Geometry: final body of the model. Coordinates: model frame, mm. Give positions to 0.01 mm unless a question says otherwise; leave off trailing zeros. Loops run counter-clockwise (first coordinate to the right, second up) from the corner with the lowest first, then second, coordinate; pieces in that order, holes last.
from build123d import *

# Parameters (mm, degrees)
SKETCH23_R          = 70.65
SKETCH23_R_2        = 14
BOSS_EXTRUDE3_DEPTH = 10
LO_BAT_HOP_SO_REACH = 12
SKETCH24_R          = 4
SKETCH24_R_2        = 6.25


with BuildPart() as part:
    # Sketch23 → Boss-Extrude3 (new body)
    with BuildSketch(Plane(origin=(0, 0, 0), x_dir=(1, 0, 0), z_dir=(0, 1, 0))):
        Polygon((106, -490.925019631), (106, 0), (79.205080757, 100), (-79.205080757, 100), (-106, 0), (-106, -490.925019631), (-20, -601), (20, -601), align=None)
        Circle(SKETCH23_R, mode=Mode.SUBTRACT)
        with Locations((0, -330)):
            Circle(SKETCH23_R_2, mode=Mode.SUBTRACT)
    extrude(amount=BOSS_EXTRUDE3_DEPTH)

    # Sketch24 → lo bat hop so (cut, up to next)
    with BuildSketch(Plane(origin=(0, 10, 0), x_dir=(1, 0, 0), z_dir=(0, 1, 0)), mode=Mode.PRIVATE) as lo_bat_hop_so_sk1:
        with Locations((-83, -150)):
            Circle(SKETCH24_R)
    lo_bat_hop_so_tool1 = extrude(lo_bat_hop_so_sk1.sketch, amount=-LO_BAT_HOP_SO_REACH, mode=Mode.PRIVATE) & part.part
    add(lo_bat_hop_so_tool1.solids().sort_by_distance((-83, 10, 150))[0], mode=Mode.SUBTRACT)
    # Sketch24 → lo bat hop so (cut, up to next)
    with BuildSketch(Plane(origin=(0, 10, 0), x_dir=(1, 0, 0), z_dir=(0, 1, 0)), mode=Mode.PRIVATE) as lo_bat_hop_so_sk2:
        with Locations((-83, -388)):
            Circle(SKETCH24_R)
    lo_bat_hop_so_tool2 = extrude(lo_bat_hop_so_sk2.sketch, amount=-LO_BAT_HOP_SO_REACH, mode=Mode.PRIVATE) & part.part
    add(lo_bat_hop_so_tool2.solids().sort_by_distance((-83, 10, 388))[0], mode=Mode.SUBTRACT)
    # Sketch24 → lo bat hop so (cut, up to next)
    with BuildSketch(Plane(origin=(0, 10, 0), x_dir=(1, 0, 0), z_dir=(0, 1, 0)), mode=Mode.PRIVATE) as lo_bat_hop_so_sk3:
        with Locations((83, -388)):
            Circle(SKETCH24_R)
    lo_bat_hop_so_tool3 = extrude(lo_bat_hop_so_sk3.sketch, amount=-LO_BAT_HOP_SO_REACH, mode=Mode.PRIVATE) & part.part
    add(lo_bat_hop_so_tool3.solids().sort_by_distance((83, 10, 388))[0], mode=Mode.SUBTRACT)
    # Sketch24 → lo bat hop so (cut, up to next)
    with BuildSketch(Plane(origin=(0, 10, 0), x_dir=(1, 0, 0), z_dir=(0, 1, 0)), mode=Mode.PRIVATE) as lo_bat_hop_so_sk4:
        with Locations((83, -150)):
            Circle(SKETCH24_R)
    lo_bat_hop_so_tool4 = extrude(lo_bat_hop_so_sk4.sketch, amount=-LO_BAT_HOP_SO_REACH, mode=Mode.PRIVATE) & part.part
    add(lo_bat_hop_so_tool4.solids().sort_by_distance((83, 10, 150))[0], mode=Mode.SUBTRACT)
    # Sketch24 → lo bat hop so (cut, up to next)
    with BuildSketch(Plane(origin=(0, 10, 0), x_dir=(1, 0, 0), z_dir=(0, 1, 0)), mode=Mode.PRIVATE) as lo_bat_hop_so_sk5:
        with Locations((-83, -20)):
            Circle(SKETCH24_R)
    lo_bat_hop_so_tool5 = extrude(lo_bat_hop_so_sk5.sketch, amount=-LO_BAT_HOP_SO_REACH, mode=Mode.PRIVATE) & part.part
    add(lo_bat_hop_so_tool5.solids().sort_by_distance((-83, 10, 20))[0], mode=Mode.SUBTRACT)
    # Sketch24 → lo bat hop so (cut, up to next)
    with BuildSketch(Plane(origin=(0, 10, 0), x_dir=(1, 0, 0), z_dir=(0, 1, 0)), mode=Mode.PRIVATE) as lo_bat_hop_so_sk6:
        with Locations((83, -20)):
            Circle(SKETCH24_R)
    lo_bat_hop_so_tool6 = extrude(lo_bat_hop_so_sk6.sketch, amount=-LO_BAT_HOP_SO_REACH, mode=Mode.PRIVATE) & part.part
    add(lo_bat_hop_so_tool6.solids().sort_by_distance((83, 10, 20))[0], mode=Mode.SUBTRACT)
    # Sketch24 → lo bat hop so (cut, up to next)
    with BuildSketch(Plane(origin=(0, 10, 0), x_dir=(1, 0, 0), z_dir=(0, 1, 0)), mode=Mode.PRIVATE) as lo_bat_hop_so_sk7:
        with Locations((-70, -380)):
            Circle(SKETCH24_R_2)
    lo_bat_hop_so_tool7 = extrude(lo_bat_hop_so_sk7.sketch, amount=-LO_BAT_HOP_SO_REACH, mode=Mode.PRIVATE) & part.part
    add(lo_bat_hop_so_tool7.solids().sort_by_distance((-70, 10, 380))[0], mode=Mode.SUBTRACT)
    # Sketch24 → lo bat hop so (cut, up to next)
    with BuildSketch(Plane(origin=(0, 10, 0), x_dir=(1, 0, 0), z_dir=(0, 1, 0)), mode=Mode.PRIVATE) as lo_bat_hop_so_sk8:
        with Locations((-70, -300)):
            Circle(SKETCH24_R_2)
    lo_bat_hop_so_tool8 = extrude(lo_bat_hop_so_sk8.sketch, amount=-LO_BAT_HOP_SO_REACH, mode=Mode.PRIVATE) & part.part
    add(lo_bat_hop_so_tool8.solids().sort_by_distance((-70, 10, 300))[0], mode=Mode.SUBTRACT)
    # Sketch24 → lo bat hop so (cut, up to next)
    with BuildSketch(Plane(origin=(0, 10, 0), x_dir=(1, 0, 0), z_dir=(0, 1, 0)), mode=Mode.PRIVATE) as lo_bat_hop_so_sk9:
        with Locations((-70, -210)):
            Circle(SKETCH24_R_2)
    lo_bat_hop_so_tool9 = extrude(lo_bat_hop_so_sk9.sketch, amount=-LO_BAT_HOP_SO_REACH, mode=Mode.PRIVATE) & part.part
    add(lo_bat_hop_so_tool9.solids().sort_by_distance((-70, 10, 210))[0], mode=Mode.SUBTRACT)
    # Sketch24 → lo bat hop so (cut, up to next)
    with BuildSketch(Plane(origin=(0, 10, 0), x_dir=(1, 0, 0), z_dir=(0, 1, 0)), mode=Mode.PRIVATE) as lo_bat_hop_so_sk10:
        with Locations((-70, -150)):
            Circle(SKETCH24_R_2)
    lo_bat_hop_so_tool10 = extrude(lo_bat_hop_so_sk10.sketch, amount=-LO_BAT_HOP_SO_REACH, mode=Mode.PRIVATE) & part.part
    add(lo_bat_hop_so_tool10.solids().sort_by_distance((-70, 10, 150))[0], mode=Mode.SUBTRACT)
    # Sketch24 → lo bat hop so (cut, up to next)
    with BuildSketch(Plane(origin=(0, 10, 0), x_dir=(1, 0, 0), z_dir=(0, 1, 0)), mode=Mode.PRIVATE) as lo_bat_hop_so_sk11:
        with Locations((-70, -90)):
            Circle(SKETCH24_R_2)
    lo_bat_hop_so_tool11 = extrude(lo_bat_hop_so_sk11.sketch, amount=-LO_BAT_HOP_SO_REACH, mode=Mode.PRIVATE) & part.part
    add(lo_bat_hop_so_tool11.solids().sort_by_distance((-70, 10, 90))[0], mode=Mode.SUBTRACT)
    # Sketch24 → lo bat hop so (cut, up to next)
    with BuildSketch(Plane(origin=(0, 10, 0), x_dir=(1, 0, 0), z_dir=(0, 1, 0)), mode=Mode.PRIVATE) as lo_bat_hop_so_sk12:
        with Locations((70, -90)):
            Circle(SKETCH24_R_2)
    lo_bat_hop_so_tool12 = extrude(lo_bat_hop_so_sk12.sketch, amount=-LO_BAT_HOP_SO_REACH, mode=Mode.PRIVATE) & part.part
    add(lo_bat_hop_so_tool12.solids().sort_by_distance((70, 10, 90))[0], mode=Mode.SUBTRACT)
    # Sketch24 → lo bat hop so (cut, up to next)
    with BuildSketch(Plane(origin=(0, 10, 0), x_dir=(1, 0, 0), z_dir=(0, 1, 0)), mode=Mode.PRIVATE) as lo_bat_hop_so_sk13:
        with Locations((70, -150)):
            Circle(SKETCH24_R_2)
    lo_bat_hop_so_tool13 = extrude(lo_bat_hop_so_sk13.sketch, amount=-LO_BAT_HOP_SO_REACH, mode=Mode.PRIVATE) & part.part
    add(lo_bat_hop_so_tool13.solids().sort_by_distance((70, 10, 150))[0], mode=Mode.SUBTRACT)
    # Sketch24 → lo bat hop so (cut, up to next)
    with BuildSketch(Plane(origin=(0, 10, 0), x_dir=(1, 0, 0), z_dir=(0, 1, 0)), mode=Mode.PRIVATE) as lo_bat_hop_so_sk14:
        with Locations((70, -210)):
            Circle(SKETCH24_R_2)
    lo_bat_hop_so_tool14 = extrude(lo_bat_hop_so_sk14.sketch, amount=-LO_BAT_HOP_SO_REACH, mode=Mode.PRIVATE) & part.part
    add(lo_bat_hop_so_tool14.solids().sort_by_distance((70, 10, 210))[0], mode=Mode.SUBTRACT)
    # Sketch24 → lo bat hop so (cut, up to next)
    with BuildSketch(Plane(origin=(0, 10, 0), x_dir=(1, 0, 0), z_dir=(0, 1, 0)), mode=Mode.PRIVATE) as lo_bat_hop_so_sk15:
        with Locations((70, -300)):
            Circle(SKETCH24_R_2)
    lo_bat_hop_so_tool15 = extrude(lo_bat_hop_so_sk15.sketch, amount=-LO_BAT_HOP_SO_REACH, mode=Mode.PRIVATE) & part.part
    add(lo_bat_hop_so_tool15.solids().sort_by_distance((70, 10, 300))[0], mode=Mode.SUBTRACT)
    # Sketch24 → lo bat hop so (cut, up to next)
    with BuildSketch(Plane(origin=(0, 10, 0), x_dir=(1, 0, 0), z_dir=(0, 1, 0)), mode=Mode.PRIVATE) as lo_bat_hop_so_sk16:
        with Locations((70, -380)):
            Circle(SKETCH24_R_2)
    lo_bat_hop_so_tool16 = extrude(lo_bat_hop_so_sk16.sketch, amount=-LO_BAT_HOP_SO_REACH, mode=Mode.PRIVATE) & part.part
    add(lo_bat_hop_so_tool16.solids().sort_by_distance((70, 10, 380))[0], mode=Mode.SUBTRACT)


solid = part.part
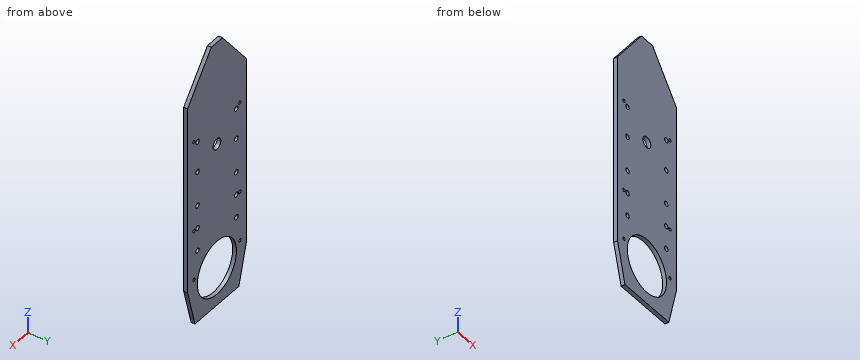
Item 1: Pin query (flat end, axial travel): pin 1 (5 mm diameter, centred on x = 83, z = 150, fed in from +Y); pin 2 (3 mm diameter, centred on x = 38.5, y = 3, fed in from +Z). Return the tip coordinate at first contact, or that it passes through.
Values follow:
pin 1: passes through
pin 2: stops at z = 579.24
Item 2: Section query A-A on z = 210. Return loops of the section in (x, y).
Values follow:
outline: (-106, 0) - (-76.25, 0) - (-76.25, 10) - (-106, 10) - close; (-63.75, 0) - (63.75, 0) - (63.75, 10) - (-63.75, 10) - close; (76.25, 0) - (106, 0) - (106, 10) - (76.25, 10) - close
Item 3: Section query B-B on z = 330. Return loops of the section in (x, y).
Values follow:
outline: (-106, 0) - (-14, 0) - (-14, 10) - (-106, 10) - close; (14, 0) - (106, 0) - (106, 10) - (14, 10) - close
Item 4: Ray query, probe 1 along X at (y, z) = (5.25, 300); probe 2 along X at (y, z) = (7, 150); probe 3 along Z at (x, y) = (-9, 5.25). Return the intervals inside material, ascending.
Values follow:
probe 1: x = -106 to -76.25, -63.75 to 63.75, 76.25 to 106
probe 2: x = -106 to -87, -79 to -76.25, -63.75 to 63.75, 76.25 to 79, 87 to 106
probe 3: z = -100 to -70.07, 70.07 to 319.28, 340.72 to 601
Item 5: Section query D-D on y = 7. Give the number of separate pieces and of enclosed holes in the cut face, plus the area to 3 significant figures.
Values follow:
separate pieces: 1
enclosed holes: 18
area: 119,000 mm2
Item 6: Section query C-C on x = 0. Return loops of the section in (y, z).
Values follow:
outline: (0, -100) - (10, -100) - (10, -70.65) - (0, -70.65) - close; (0, 70.65) - (10, 70.65) - (10, 316) - (0, 316) - close; (0, 344) - (10, 344) - (10, 601) - (0, 601) - close
